Can you work these out from the model? Positions are in its coordinate system, mm. A direction names the side the tool comes from. Coordinates: 2 decimals unless noted, no trailing zeros. Loops run counter-clockwise (first coordinate to the right, second up) from the corner with the lowest first, then second, coordinate; pieces in that order, holes last. Notation, with made-up numbers: (8, -38) -> (38, -38) arc R9 ccw to (38, -34) -> close; hole circle Ø6 at (-32.75, 30.25). An arc over 180 degrees is marked (long way). Put each result on its own line as item: value. Start each with the question number.
Item 1: Will these pins go through, and if not, where does the flat tip stop? P1, Ø1.2, axis at x = -0.5, y = 0.5, coming from the -Z side; P2, Ø2, axis at x = -0.5, z = 6, coming from the -Y side (3 decimals); P3, Ø1.6, axis at x = -0.5, z = 6, coming from the +Y side (3 decimals).
Item 2: If we section it at B-B on z = 1: Please give me the cut outline in (x, y), plus the area to 3 significant figures.
Item 3: If we section it at D-D on z = 6: Please give me the cut outline in (x, y) (3 decimals), plus the area to 3 significant figures.
Item 4: For faces 4 (the flat face through (-1.425, 0, 4)), 5 (the flat face through (0, -1.925, 6)), 6 (the flat face through (0, 2.05, 2)), 7 (the flat face through (-1.925, 0, 6)), which set-ups out of +Z, -Z, +X, -X, +Y, -Y let a thin tool reach every point of the face, with its end or its side?
Item 5: Please list where these lines run through material, in increasing order: L1, parallel to Z at x = 0, y = 4.75; L2, parallel to Y at x = 0.75, z = 4 (3 decimals); L3, parallel to X at y = 1.25, z = 1. Write a range as from..to.
Item 6: We'd pull the mould along Y, two halves only. Please class faces 1 (the flat face through (0, -2.05, 2)), 2 (the flat face through (0, -1.425, 4)), 3 (the flat face through (1.425, 0, 4)): pulls with the +Y half, pulls with the -Y half, needs draft (parallel to the pull), parting line crosses it, or undercut.
Item 7: If we section it at A-A on x = 0: Please give me the cut outline in (y, z) (3 decimals).
Autodesk Fusion 360 part; units mm, degrees
sketch "Sketch1" plane through (0, 0, 0) normal (0, 0, 1) x (1, 0, 0)
  circle A0 centre (0, 0) radius 5.75
  line L0 (1.925, -1.925) -> (-1.925, -1.925)
  line L1 (-1.925, -1.925) -> (-1.925, 1.925)
  line L2 (-1.925, 1.925) -> (1.925, 1.925)
  line L3 (1.925, 1.925) -> (1.925, -1.925)
  line L4 (1.925, -1.925) -> (-1.925, 1.925) construction
  line L5 (-1.925, -1.925) -> (1.925, 1.925) construction
  line L6 (-1.425, 1.425) -> (1.425, 1.425)
  line L7 (1.425, 1.425) -> (1.425, -1.425)
  line L8 (1.425, -1.425) -> (-1.425, -1.425)
  line L9 (-1.425, -1.425) -> (-1.425, 1.425)
  line L10 (-2.05, -2.05) -> (2.05, -2.05)
  line L11 (2.05, -2.05) -> (2.05, 2.05)
  line L12 (2.05, 2.05) -> (-2.05, 2.05)
  line L13 (-2.05, 2.05) -> (-2.05, -2.05)
  line L14 (-2.05, -2.05) -> (2.05, 2.05) construction
  line L15 (2.05, -2.05) -> (-2.05, 2.05) construction
  dimension "d1" = 11.5
  dimension "d2" = 3.85
  dimension "d3" = 3.85
  dimension "d11" = 0.5
  dimension "d12" = 4.1
  dimension "d13" = 4.1
extrude "Extrude1" add sketch "Sketch1" along normal blind 3.7 contours A0 | L0 L1 L2 L3 | L6 L7 L8 L9 | L10 L11 L12 L13
extrude "Extrude2" cut sketch "Sketch1" along normal blind 3.1 contours L0 L1 L2 L3 | L6 L7 L8 L9 | L10 L11 L12 L13
extrude "Extrude3" add sketch "Sketch1" along normal blind 3 from surface at 3.7 contours L0 L1 L2 L3 | L6 L7 L8 L9
extrude "Extrude4" cut sketch "Sketch1" along normal blind 1 from surface at 3.7 contours L0 L1 L2 L3 | L10 L11 L12 L13
Solutions:
1. P1: z = 3.1
1. P2: y = -1.925
1. P3: y = 1.925
2. outline: circle Ø11.5 at (0, 0); hole (-2.05, -2.05) -> (2.05, -2.05) -> (2.05, 2.05) -> (-2.05, 2.05) -> close
2. area: 87.1 mm^2
3. outline: (-1.925, -1.925) -> (1.925, -1.925) -> (1.925, 1.925) -> (-1.925, 1.925) -> close
3. area: 14.8 mm^2
4. face 4: -X, +Y, -Y
4. face 5: +Z, +X, -X, -Y
4. face 6: -Z
4. face 7: +Z, -X, +Y, -Y
5. L1: 0..3.7
5. L2: -1.425..1.425
5. L3: -5.61..-2.05, 2.05..5.61
6. face 1: undercut
6. face 2: pulls with the -Y half
6. face 3: needs draft
7. outline: (-5.75, 0) -> (-2.05, 0) -> (-2.05, 3.1) -> (2.05, 3.1) -> (2.05, 0) -> (5.75, 0) -> (5.75, 3.7) -> (1.425, 3.7) -> (1.425, 4.7) -> (1.925, 4.7) -> (1.925, 6.7) -> (-1.925, 6.7) -> (-1.925, 4.7) -> (-1.425, 4.7) -> (-1.425, 3.7) -> (-5.75, 3.7) -> close
